```python
from build123d import *

# Parameters (mm, degrees)
SKETCH1_W               = 302
SKETCH1_H               = 394
BOSS_EXTRUDE1_DEPTH     = 1
CUT_EXTRUDE2_DEPTH      = 249.215632062
MIRROR2_COPY_1_DEPTH    = 249.215632062
SKETCH4_R               = 1.5
CUT_EXTRUDE3_DEPTH      = 249.215632062
MIRROR4_COPY_1_SKETCH_R = 1.5
MIRROR4_COPY_1_DEPTH    = 249.215632062
SKETCH5_W               = 120
SKETCH5_H               = 42.5
CUT_EXTRUDE4_DEPTH      = 249.215632062


with BuildPart() as part:
    # Sketch1 → Boss-Extrude1 (new body)
    with BuildSketch(Plane(origin=(0, 0, 0), x_dir=(1, 0, 0), z_dir=(0, 1, 0))):
        Rectangle(SKETCH1_W, SKETCH1_H)
    extrude(amount=BOSS_EXTRUDE1_DEPTH)

    # Sketch3 → Cut-Extrude2 (cut, through all)
    with BuildSketch(Plane(origin=(0, 1, 0), x_dir=(1, 0, 0), z_dir=(0, 1, 0))):
        with BuildLine():
            Line((-151, 147), (-101, 147))
            ThreePointArc((-101, 147), (-100.5, 146.5), (-101, 146))
            Line((-101, 146), (-151, 146))
            ThreePointArc((-151, 146), (-151.5, 146.5), (-151, 147))
        make_face()
    cut_extrude2 = extrude(amount=-CUT_EXTRUDE2_DEPTH, mode=Mode.SUBTRACT)

    # Mirror1: Cut-Extrude2 across plane
    add(cut_extrude2.mirror(Plane.XY), mode=Mode.SUBTRACT)

    # Mirror2: Cut-Extrude2 across plane
    add(cut_extrude2.mirror(Plane(origin=(0, 0, 0), x_dir=(0, 0, 1), z_dir=(1, 0, 0))), mode=Mode.SUBTRACT)

    # Mirror2 copy 1 sketch → Mirror2 copy 1 (cut, through all)
    with BuildSketch(Plane(origin=(0, 1, 0), x_dir=(-1, 0, 0), z_dir=(0, 1, 0))):
        with BuildLine():
            Line((-151, 147), (-101, 147))
            ThreePointArc((-101, 147), (-100.5, 146.5), (-101, 146))
            Line((-101, 146), (-151, 146))
            ThreePointArc((-151, 146), (-151.5, 146.5), (-151, 147))
        make_face()
    extrude(amount=-MIRROR2_COPY_1_DEPTH, mode=Mode.SUBTRACT)

    # Sketch4 → Cut-Extrude3 (cut, through all)
    with BuildSketch(Plane(origin=(0, 1, 0), x_dir=(1, 0, 0), z_dir=(0, 1, 0))):
        with Locations(Location((-111, 91, 0), (0, 0, 270))):
            Circle(SKETCH4_R)
    cut_extrude3 = extrude(amount=-CUT_EXTRUDE3_DEPTH, mode=Mode.SUBTRACT)

    # Mirror3: Cut-Extrude3 across plane
    add(cut_extrude3.mirror(Plane(origin=(0, 0, 0), x_dir=(0, 0, 1), z_dir=(1, 0, 0))), mode=Mode.SUBTRACT)

    # Mirror4: Cut-Extrude3 across plane
    add(cut_extrude3.mirror(Plane.XY), mode=Mode.SUBTRACT)

    # Mirror4 copy 1 sketch → Mirror4 copy 1 (cut, through all)
    with BuildSketch(Plane(origin=(0, 1, 0), x_dir=(-1, 0, 0), z_dir=(0, 1, 0))):
        with Locations(Location((-111, 91, 0), (0, 0, 270))):
            Circle(MIRROR4_COPY_1_SKETCH_R)
    extrude(amount=-MIRROR4_COPY_1_DEPTH, mode=Mode.SUBTRACT)

    # Sketch5 → Cut-Extrude4 (cut, through all)
    with BuildSketch(Plane(origin=(0, 1, 0), x_dir=(1, 0, 0), z_dir=(0, 1, 0))):
        with Locations((0, 175.75)):
            Rectangle(SKETCH5_W, SKETCH5_H)
    extrude(amount=-CUT_EXTRUDE4_DEPTH, mode=Mode.SUBTRACT)


solid = part.part
```
Here's how the part is built. I have some questions about the finished solid (model axes, mm). Round coordinates to 2 decimals unless told otherwise and drop trailing zeros. Loops run counter-clockwise (first coordinate to the right, second up) from the corner with the lowest first, then second, coordinate; pieces in that order, holes last.
1. Will these pins go through, and if not, where does the flat tip stop? pin 1 (8 mm diameter, centred on x = -90.5, z = 66, fed in from -Y); pin 2 (0.5 mm diameter, centred on x = -23.5, y = 0.5, fed in from -Z).
Answers:
pin 1: stops at y = 0
pin 2: stops at z = -154.5
2. Suppose I cut it at A-A, the plane y = 0.3. Please give me the cut outline in (x, z), and give its area (3 significant figures).
Answers:
outline: (-151, -197) - (-60, -197) - (-60, -154.5) - (60, -154.5) - (60, -197) - (151, -197) - (151, -147) - (101, -147) arc R0.5 cw to (101, -146) - (151, -146) - (151, 146) - (101, 146) arc R0.5 cw to (101, 147) - (151, 147) - (151, 197) - (-151, 197) - (-151, 147) - (-101, 147) arc R0.5 cw to (-101, 146) - (-151, 146) - (-151, -146) - (-101, -146) arc R0.5 cw to (-101, -147) - (-151, -147) - close; hole circle Ø3 at (-111, -91); hole circle Ø3 at (-111, 91); hole circle Ø3 at (111, -91); hole circle Ø3 at (111, 91)
area: 114,000 mm2
3. If I drill on probe 1 along Z at (x, y) = (126, 0.9); probe 2 along X at (y, z) = (0.4, 91); probe 3 along Z at (x, y) = (-111, 0.85), over which ranges is the centre line in solid material (lowest first)?
Answers:
probe 1: z = -197 to -147, -146 to 146, 147 to 197
probe 2: x = -151 to -112.5, -109.5 to 109.5, 112.5 to 151
probe 3: z = -197 to -147, -146 to -92.5, -89.5 to 89.5, 92.5 to 146, 147 to 197
4. Thinking about a two-plate mould opening in Y: for faces 1 (the face through (-2, 0, -3)), 2 (the face through (-2, 1, -3)), which applies, released by +Y, released by -Y, zero draft, split by the parting line, or undercut?
Answers:
face 1: released by -Y
face 2: released by +Y
